Work out the finished part from the listing and answer in its coordinate system (mm). A direction names the side the tool comes from. Coordinates: 2 decimals unless noted, no trailing zeros. Order: outer loops, then holes, each group sorted by start corner. A loop starts at its lowest first (then second) coordinate and runs counter-clockwise, first axis right, second up.
1. The part is cut by section C-C, the plane y = 10. Give the vertices of the cut face in (x, z).
2. Flat-ended cylindrical pins translate along their axes: pin 1 Ø4 at (x, y) = (18.5, 17) entering from +Z; pin 2 Ø5 at (x, y) = (10, 26) entering from -Z; pin 3 Ø8 at (y, z) = (12, 10.5) entering from +X; pin 4 Ø1.5 at (y, z) = (29, 2.5) entering from +X. Find the tip coordinate at first contact, or state that the pin passes through.
3. A tool of negligible diameter and unlimited length cuts with its end or side. For faces 4 (the flat face through (33, 10, 2)), 5 (the flat face through (27.3, 8.7, 3)), 6 (the flat face through (20, 26, 2)), from which of +Z, -Z, +X, -X, +Y, -Y can it reach the whole face along a straight path? Write none if from no direction.
4. The part is cut by section A-A, the plane y = 26. Give the vertices of the cut face in (x, z).
5. Find the intervals of material crossed by probe 1 along Y at (x, z) = (10, 3.75); probe 2 along Y at (x, z) = (10, 2.4); probe 3 along Y at (x, z) = (26, 1), in increasing order.
6. Determine the mould class of faces 1 (the flat face through (16, 0, 2)), 2 (the flat face through (13, 17, 0)), 3 (the cylindrical face through (8.82, 27.08, 1.48)) for opening direction Y: +Y half, -Y half, draft (parallel to the pull), parting line (faces both ways), or undercut.
```python
from build123d import *

# Parameters (mm, degrees)
SKETCH_1_W          = 20
SKETCH_1_H          = 20
SKETCH_1_H_2        = 13
SKETCH_1_R          = 1.6
SKETCH_1_W_2        = 13
EXTRUDE_1_DEPTH     = 5
SKETCH_2_R          = 6
EXTRUDE_2_DEPTH     = 10
SKETCH_3_R          = 2.4
CUT_EXTRUDE_1_DEPTH = 50.020403915
SKETCH_4_R          = 3
CUT_EXTRUDE_2_DEPTH = 2
FILLET_1_R          = 0.5


with BuildPart() as part:
    # 草图1 → 凸台-拉伸1 (new body)
    # profile 1 of 3: a face of its own
    with BuildSketch(Plane.XY):
        with Locations((10, 10)):
            Rectangle(SKETCH_1_W, SKETCH_1_H)
    # profile 2 of 3: a face of its own
    with BuildSketch(Plane.XY):
        with Locations((10, 26.5)):
            Rectangle(SKETCH_1_W, SKETCH_1_H_2)
        with Locations((10, 26)):
            Circle(SKETCH_1_R, mode=Mode.SUBTRACT)
    # profile 3 of 3: a face of its own
    with BuildSketch(Plane.XY):
        with Locations((26.5, 10)):
            Rectangle(SKETCH_1_W_2, SKETCH_1_H)
        with Locations((26, 10)):
            Circle(SKETCH_1_R, mode=Mode.SUBTRACT)
    extrude(amount=EXTRUDE_1_DEPTH)

    # 草图2 → 凸台-拉伸2 (add)
    with BuildSketch(Plane.XY.offset(5)):
        with Locations((10, 10)):
            Circle(SKETCH_2_R)
    extrude(amount=EXTRUDE_2_DEPTH)

    # 草图3 → 切除-拉伸1 (cut, through all)
    with BuildSketch(Plane.XY.offset(15)):
        with Locations((10, 10)):
            Circle(SKETCH_3_R)
    extrude(amount=-CUT_EXTRUDE_1_DEPTH, mode=Mode.SUBTRACT)

    # 草图4 → 切除-拉伸2 (cut)
    with BuildSketch(Plane.XY.offset(5)):
        with Locations((10, 26)):
            Circle(SKETCH_4_R)
        with Locations((26, 10)):
            Circle(SKETCH_4_R)
    extrude(amount=-CUT_EXTRUDE_2_DEPTH, mode=Mode.SUBTRACT)

    # 圆角1
    fillet_1_edges = [part.edges().sort_by_distance(p)[0] for p in [
        (7.6, 10, 15),
    ]]
    fillet(fillet_1_edges, radius=FILLET_1_R)


solid = part.part
```
Geometry says:
1. outline: (0, 0) - (7.6, 0) - (7.6, 14.5) arc R0.5 ccw to (7.1, 15) - (4, 15) - (4, 5) - (0, 5) - close; (12.4, 0) - (24.4, 0) - (24.4, 3) - (23, 3) - (23, 5) - (16, 5) - (16, 15) - (12.9, 15) arc R0.5 ccw to (12.4, 14.5) - close; (27.6, 0) - (33, 0) - (33, 5) - (29, 5) - (29, 3) - (27.6, 3) - close
2. pin 1: stops at z = 5
2. pin 2: stops at z = 0
2. pin 3: stops at x = 16
2. pin 4: stops at x = 20
3. face 4: +Z, -Z, +X, +Y, -Y
3. face 5: +Z
3. face 6: +Z, -Z, +X, +Y
4. outline: (0, 0) - (8.4, 0) - (8.4, 3) - (7, 3) - (7, 5) - (0, 5) - close; (11.6, 0) - (20, 0) - (20, 5) - (13, 5) - (13, 3) - (11.6, 3) - close
5. probe 1: y = 0 to 7.6, 12.4 to 23, 29 to 33
5. probe 2: y = 0 to 7.6, 12.4 to 24.4, 27.6 to 33
5. probe 3: y = 0 to 8.4, 11.6 to 20
6. face 1: -Y half
6. face 2: draft
6. face 3: undercut
